from build123d import *

# Parameters (mm, degrees)
BOSS_EXTRUDE1_DEPTH = 3.175
SKETCH2_R           = 14.2875
CUT_EXTRUDE1_DEPTH  = 4.175
SKETCH4_R           = 6.35
SKETCH4_R_2         = 3.175
CUT_EXTRUDE2_DEPTH  = 4.175
SKETCH8_R           = 9.779
BOSS_EXTRUDE3_DEPTH = 3.175
SKETCH9_R           = 2.0193
CUT_EXTRUDE3_DEPTH  = 4.175
SKETCH10_W          = 38.1
SKETCH10_H          = 100.0125
CUT_EXTRUDE4_DEPTH  = 4.175
CUT_EXTRUDE5_DEPTH  = 4.175


with BuildPart() as part:
    # Sketch1 → Boss-Extrude1 (new body)
    with BuildSketch(Plane.XY):
        with BuildLine():
            Line((-35.603982701, 119.957272705), (-127, -119.957272705))
            Line((-127, -119.957272705), (127, -119.957272705))
            Line((127, -119.957272705), (35.603982701, 119.957272705))
            ThreePointArc((35.603982701, 119.957272705), (0, 144.493850724), (-35.603982701, 119.957272705))
        make_face()
    extrude(amount=BOSS_EXTRUDE1_DEPTH)

    # Sketch2 → Cut-Extrude1 (cut, through all)
    with BuildSketch(Plane.XY.offset(3.175)):
        with Locations((0, 106.393850724)):
            Circle(SKETCH2_R)
    extrude(amount=-CUT_EXTRUDE1_DEPTH, mode=Mode.SUBTRACT)

    # Sketch4 → Cut-Extrude2 (cut, through all)
    with BuildSketch(Plane.XY.offset(3.175)):
        with Locations((108.571571229, -107.257272705)):
            Circle(SKETCH4_R)
        with Locations((-76.2, -107.257272705)):
            Circle(SKETCH4_R_2)
        with Locations((19.05, -107.257272705)):
            Circle(SKETCH4_R_2)
    extrude(amount=-CUT_EXTRUDE2_DEPTH, mode=Mode.SUBTRACT)

    # Sketch8 → Boss-Extrude3 (add)
    with BuildSketch(Plane(origin=(0, 0, 0), x_dir=(-1, 0, 0), z_dir=(0, 0, -1))):
        with BuildLine():
            Line((-127, -119.957272705), (-183.251300865, -119.957272705))
            ThreePointArc((-183.251300865, -119.957272705), (-218.176300865, -85.032272705), (-183.251300865, -50.107272705))
            Line((-183.251300865, -50.107272705), (-100.39047619, -50.107272705))
            Line((-100.39047619, -50.107272705), (-127, -119.957272705))
        make_face()
        with Locations((-183.251300865, -85.032272705)):
            Circle(SKETCH8_R, mode=Mode.SUBTRACT)
    extrude(amount=-BOSS_EXTRUDE3_DEPTH)

    # Sketch9 → Cut-Extrude3 (cut, through all)
    with BuildSketch(Plane.XY.offset(3.175)):
        with Locations((183.251300865, -59.632272705)):
            Circle(SKETCH9_R)
        with Locations((183.251300865, -110.432272705)):
            Circle(SKETCH9_R)
    extrude(amount=-CUT_EXTRUDE3_DEPTH, mode=Mode.SUBTRACT)

    # Sketch10 → Cut-Extrude4 (cut, through all)
    with BuildSketch(Plane.XY.offset(3.175)):
        with Locations((-107.95, -69.951022705)):
            Rectangle(SKETCH10_W, SKETCH10_H)
    extrude(amount=-CUT_EXTRUDE4_DEPTH, mode=Mode.SUBTRACT)

    # Sketch11 → Cut-Extrude5 (cut, through all)
    with BuildSketch(Plane.XY.offset(3.175)):
        with BuildLine():
            Line((-34.41372286, 69.569766501), (-61.423985812, -1.332173746))
            ThreePointArc((-61.423985812, -1.332173746), (-60.365933576, -10.128014274), (-52.522990136, -14.248029241))
            Line((-52.522990136, -14.248029241), (-19.05, -14.248029241))
            ThreePointArc((-19.05, -14.248029241), (-12.314807909, -11.458221332), (-9.525, -4.723029241))
            Line((-9.525, -4.723029241), (-9.525, 62.74481723))
            ThreePointArc((-9.525, 62.74481723), (-11.080813247, 67.96187459), (-15.24, 71.474623928))
            ThreePointArc((-15.24, 71.474623928), (-17.877940169, 72.748802718), (-20.410181748, 74.221898949))
            ThreePointArc((-20.410181748, 74.221898949), (-28.515665768, 75.218157925), (-34.41372286, 69.569766501))
        make_face()
        with BuildLine():
            Line((19.05, -14.248029241), (52.522990136, -14.248029241))
            ThreePointArc((52.522990136, -14.248029241), (60.365933576, -10.128014274), (61.423985812, -1.332173746))
            Line((61.423985812, -1.332173746), (34.41372286, 69.569766501))
            ThreePointArc((34.41372286, 69.569766501), (28.515665768, 75.218157925), (20.410181748, 74.221898949))
            ThreePointArc((20.410181748, 74.221898949), (17.877940169, 72.748802718), (15.24, 71.474623928))
            ThreePointArc((15.24, 71.474623928), (11.080813247, 67.96187459), (9.525, 62.74481723))
            Line((9.525, 62.74481723), (9.525, -4.723029241))
            ThreePointArc((9.525, -4.723029241), (12.314807909, -11.458221332), (19.05, -14.248029241))
        make_face()
        with BuildLine():
            Line((-19.05, -33.298029241), (-60.325, -33.298029241))
            ThreePointArc((-60.325, -33.298029241), (-67.060192091, -36.087837151), (-69.85, -42.823029241))
            Line((-69.85, -42.823029241), (-69.85, -72.332272705))
            ThreePointArc((-69.85, -72.332272705), (-67.060192091, -79.067464796), (-60.325, -81.857272705))
            Line((-60.325, -81.857272705), (-19.05, -81.857272705))
            ThreePointArc((-19.05, -81.857272705), (-12.314807909, -79.067464796), (-9.525, -72.332272705))
            Line((-9.525, -72.332272705), (-9.525, -42.823029241))
            ThreePointArc((-9.525, -42.823029241), (-12.314807909, -36.087837151), (-19.05, -33.298029241))
        make_face()
        with BuildLine():
            Line((9.525, -42.823029241), (9.525, -72.332272705))
            ThreePointArc((9.525, -72.332272705), (12.314807909, -79.067464796), (19.05, -81.857272705))
            Line((19.05, -81.857272705), (78.278892408, -81.857272705))
            ThreePointArc((78.278892408, -81.857272705), (86.121835848, -77.737257738), (87.179888084, -68.94141721))
            Line((87.179888084, -68.94141721), (75.938271526, -39.432173746))
            ThreePointArc((75.938271526, -39.432173746), (72.442260883, -34.980085802), (67.037275851, -33.298029241))
            Line((67.037275851, -33.298029241), (19.05, -33.298029241))
            ThreePointArc((19.05, -33.298029241), (12.314807909, -36.087837151), (9.525, -42.823029241))
        make_face()
    extrude(amount=-CUT_EXTRUDE5_DEPTH, mode=Mode.SUBTRACT)


solid = part.part
Read the model definition and answer for the solid it produces. Units are mm, in the model's axes. A direction names the side the tool comes from. Round coordinates to 2 decimals unless told otherwise and drop trailing zeros. Write each loop counter-clockwise with the first axis right and the second up, starting at its lowest first coordinate (ties: lowest second). Pieces come first, ordered by that corner, then holes. Notation, with made-up numbers: M 48,62.25 L 101,62.25 A29 cw 101,98.25 Z; hole C 77.5,-19 d2. An arc over 180 degrees is marked long. Use a Markdown table: item, result.
1) For a pull along Y with two mould halves and no side action, classify faces 3 (the cylindrical face through (218.168, -85.8, 1.565)), 4 (the cylindrical face through (-66.986, -36.014, 1.61)), 5 (the flat face through (28, -15, 0)), 6 (the cylindrical face through (-1.86, 120.56, 1.61)) as pulls with the +Y half, pulls with the -Y half, needs draft (parallel to the pull), parting line crosses it, or undercut.
Answers follow:
| item | result |
|---|---|
| face 3 | parting line crosses it |
| face 4 | undercut |
| face 5 | needs draft |
| face 6 | undercut |
2) Flat-ended cylindrical pins translate along their axes: pin 1 (1.6 mm diameter, centred on y = 30.5, z = 2, fed in from +X); pin 2 (1.5 mm diameter, centred on y = -0.5, z = 2.5, fed in from +X); pin 3 (1.6 mm diameter, centred on x = 34, z = 2, fed in from +Y). Find the tip coordinate at first contact, or state that the pin passes through.
Answers follow:
| item | result |
|---|---|
| pin 1 | stops at x = 69.99 |
| pin 2 | stops at x = 81.78 |
| pin 3 | stops at y = 125.09 |
3) The part is cut by section D-D (z = 1.4). Give the number of separate pieces and of enclosed holes in the cut face, plus the area to 3 significant figures.
Answers follow:
| item | result |
|---|---|
| separate pieces | 1 |
| enclosed holes | 11 |
| area | 30,800 mm2 |
4) The part is cut by section C-C (x = 130). Write down the section's boundary in (y, z) (3 decimals).
Answers follow:
| item | result |
|---|---|
| outline | M -119.957,0 L -50.107,0 L -50.107,3.175 L -119.957,3.175 Z |
5) The part is cut by section B-B (y = 20). Write down the section's boundary in (x, z) (3 decimals).
Answers follow:
| item | result |
|---|---|
| outline | M -73.683,0 L -53.297,0 L -53.297,3.175 L -73.683,3.175 Z; M -9.525,0 L 9.525,0 L 9.525,3.175 L -9.525,3.175 Z; M 53.297,0 L 73.683,0 L 73.683,3.175 L 53.297,3.175 Z |
6) A tool of negligible diameter and unlimited length cuts with its end or side. For faces 1 (the flat face through (68.451, 33.735, 1.565)), 2 (the cylindrical face through (-67.134, -78.993, 1.61)), from which of +Z, -Z, +X, -X, +Y, -Y can it reach the whole face along a straight path? Write none if from no direction.
Answers follow:
| item | result |
|---|---|
| face 1 | +Z, -Z, +X, +Y |
| face 2 | +Z, -Z |
7) The part is cut by section A-A (x = 0). Write down the section's boundary in (y, z) (3 decimals), plus the area to 3 significant figures.
Answers follow:
| item | result |
|---|---|
| outline | M -119.957,0 L 92.106,0 L 92.106,3.175 L -119.957,3.175 Z; M 120.681,0 L 144.494,0 L 144.494,3.175 L 120.681,3.175 Z |
| area | 749 mm2 |
8) Straight lines are drawn through the part: line 1 along X through (y, z) = (-36.5, 1.35); line 2 along X through (y, z) = (52, 2.9) (3 decimals); line 3 along Y through (x, z) = (-19, 2.4). For each, find the intervals that lie inside material, in ascending order. Write a range as [from, to].
Answers follow:
| item | result |
|---|---|
| line 1 | x = [-88.9, -67.45], [-11.93, 11.93], [74.16, 95.21] |
| line 2 | x = [-61.492, -41.107], [-9.525, 9.525], [41.107, 61.492] |
| line 3 | y = [-119.96, -81.86], [-33.3, -14.25], [73.37, 139.42] |
